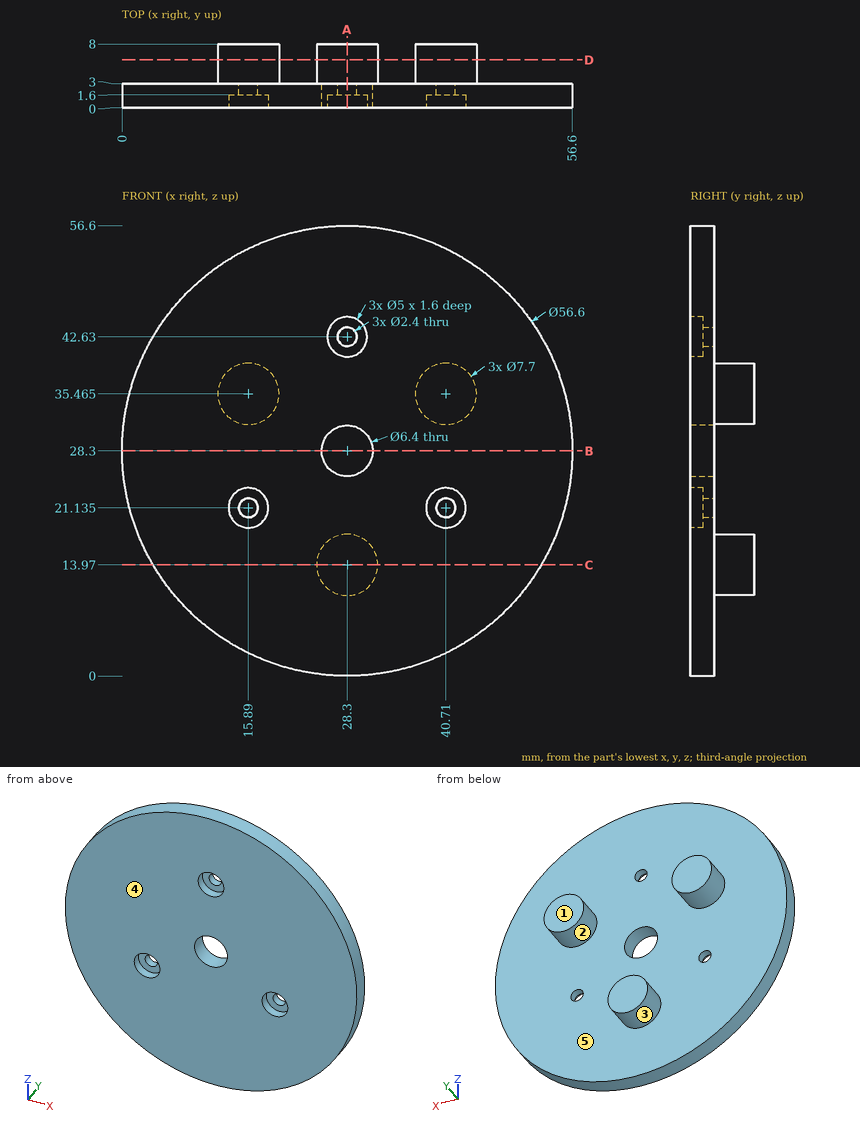
Answer from the drawing. Dimensions are ordinates in mm from the lowest x, y and z of the part. A direction names the side the tool comes from. Round coordinates to 2 decimals unless told otherwise and drop trailing zeros. Write each loop counter-clockwise with the first axis right and the second up, starting at its lowest first coordinate (ties: lowest second). Pieces come first, ordered by that corner, then holes. Notation, with made-up numbers: (8, 71.5) -> (18, 71.5) arc R26 cw to (18, 107.5) -> close; hole circle Ø1 at (-35.75, -32). An arc over 180 degrees is marked (long way). Answer in a Markdown table with one row per item. Add a question column.
1) Find section C-C, the plane z = 13.97. Determine the outline of the cut face in (x, y).
2) Find section D-D, the plane y = 6. Determine the outline of the cut face in (x, z) (3 decimals).
3) Given P1, Ø1.5, axis at x = 42.5, y = 5, coming from the +Z side; P2, Ø4, axis at x = 28.3, z = 42.63, coming from the -Y side; P3, Ø1, axis at x = 14, z = 29, coming from the +Y side, each flat-ended and moving along its own axis, determine where each tip first touches the part or whether it passes through.
4) Consider line 1 (Y direction, x = 37, z = 5); line 2 (X direction, y = 1.75, z = 30); line 3 (X direction, y = 1, z = 26) (1 decimal). Determine where each line is inside the solid, lowest interval first.
5) Find section B-B, the plane z = 28.3. Determine the outline of the cut face in (x, y).
6) Determine the mould class of the marked faces 1, 2 and 3 for opening direction X: pulls with the +X half, pulls with the -X half, needs draft (parallel to the pull), parting line crosses it, or undercut.
7) Find section A-A, the plane x = 28.3. Determine the outline of the cut face in (y, z).
8) Which of the six approach directions +Z, -Z, +X, -X, +Y, -Y give full straight-line access (tool end or side, diameter ignored) to the marked faces 4 and 5?
Findings below:
| question | item | result |
|---|---|---|
| 1 | outline | (3.9, 0) -> (52.7, 0) -> (52.7, 3) -> (32.15, 3) -> (32.15, 8) -> (24.45, 8) -> (24.45, 3) -> (3.9, 3) -> close |
| 2 | outline | circle Ø7.7 at (15.89, 35.465); circle Ø7.7 at (28.3, 13.97); circle Ø7.7 at (40.71, 35.465) |
| 3 | P1 | z = 39.17 |
| 3 | P2 | y = 1.6 |
| 3 | P3 | y = 3 |
| 4 | line 1 | 0 to 3 |
| 4 | line 2 | 0.05 to 25.59, 31.01 to 56.55 |
| 4 | line 3 | 0.1 to 26.1, 30.5 to 56.5 |
| 5 | outline | (0, 0) -> (25.1, 0) -> (25.1, 3) -> (0, 3) -> close; (31.5, 0) -> (56.6, 0) -> (56.6, 3) -> (31.5, 3) -> close |
| 6 | face 1 | needs draft |
| 6 | face 2 | undercut |
| 6 | face 3 | parting line crosses it |
| 7 | outline | (0, 0) -> (3, 0) -> (3, 10.12) -> (8, 10.12) -> (8, 17.82) -> (3, 17.82) -> (3, 25.1) -> (0, 25.1) -> close; (0, 31.5) -> (3, 31.5) -> (3, 41.43) -> (1.6, 41.43) -> (1.6, 40.13) -> (0, 40.13) -> close; (0, 45.13) -> (1.6, 45.13) -> (1.6, 43.83) -> (3, 43.83) -> (3, 56.6) -> (0, 56.6) -> close |
| 8 | face 4 | +Z, -Z, +X, -X, -Y |
| 8 | face 5 | +Y |
